Design review of the part built by this model. Coordinates are the model's own, in mm. Face numbers are marked on the shaded views. A direction names the side the tool comes from. Coordinates: 2 decimals unless noted, no trailing zeros. Loops run counter-clockwise (first coordinate to the right, second up) from the corner with the lowest first, then second, coordinate; pieces in that order, holes last. Notation, with made-up numbers: M 34,46 L 72,46 A24 cw 72,66 Z; hole C 61.25,-12 d10. An arc over 180 degrees is marked long. Put each result on its own line as item: value. Start each with the question number.
(1) For probe 1 along Z at (x, y) = (-14, -17.15); probe 2 along X at (y, z) = (-17.15, 0); probe 3 along X at (y, z) = (-19.5, -2.5), list the stretches that pass through material, from the lowest coordinate up. Write a range as [from, to].
(2) Take a section at D-D, the plane x = -5.5. Give the boundary of the cut face in (y, z), then the cut area to 3 significant figures.
(3) Clearance check with flat-ended pins moving along their axes: pin 1 (1.5 mm diameter, centred on x = 13, z = 2, fed in from +Y); pin 2 (1.6 mm diameter, centred on x = -14, z = 0, fed in from +Y); pin 3 (6.5 mm diameter, centred on y = -9.5, z = -0.5, fed in from -X); pin 4 (4 mm diameter, centred on y = -21, z = -1, fed in from +X). State where each tip first meets the part, or that it passes through.
(4) For the marked faces 1, 2, 3, 4 and 5, list the 3-axis set-ups (+Z, -Z, +X, -X, +Y, -Y) from which the entire face can be reached by the end or side of a thin tool; tool diameter is ignored.
(5) Take a section at C-C, the plane z = 2. Give the boundary of the cut face in (x, y).
(6) Take a section at B-B, the plane y = -16.25. Give the boundary of the cut face in (x, z), then the cut area to 3 significant figures.
(7) Take a section at A-A, the plane x = 14. Give the boundary of the cut face in (y, z).
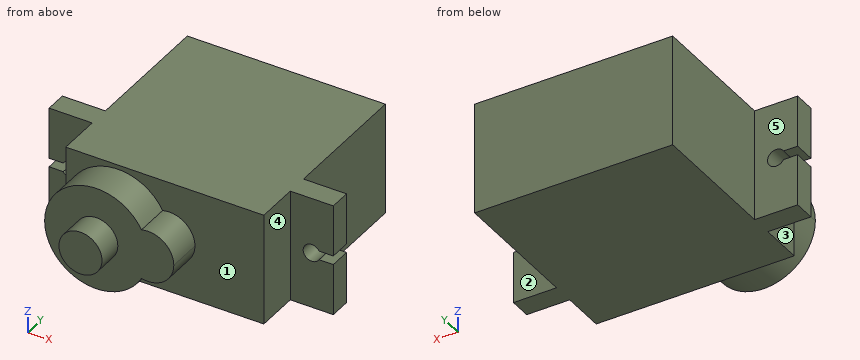
```python
from build123d import *

# Parameters (mm, degrees)
F0_R     = 2.5
F1_DEPTH = 23
F2_START = 15.5
F2_DEPTH = 2.5
F4_START = 23
F4_DEPTH = 4
F5_DEPTH = 30


with BuildPart() as f1:
    # F0 (on Front) → F1 (new body)
    with BuildSketch(Plane.XZ):
        Polygon((-11.5, -6.5), (11.5, -6.5), (11.5, 6.5), (-11.5, 6.5), (-11.5, 0), align=None)
        with BuildLine():
            ThreePointArc((-0.25, -2.9047375097), (-7, -5.8094750193), (-11.5, 0))
            ThreePointArc((-11.5, 0), (-7, 5.8094750193), (-0.25, 2.9047375097))
            ThreePointArc((-0.25, 2.9047375097), (2.3371173071, 2.3717082451), (3.5, 0))
            ThreePointArc((3.5, 0), (2.3371173071, -2.3717082451), (-0.25, -2.9047375097))
        make_face(mode=Mode.SUBTRACT)
        with BuildLine():
            ThreePointArc((3.5, 0), (2.3371173071, 2.3717082451), (-0.25, 2.9047375097))
            ThreePointArc((-0.25, 2.9047375097), (0.3094750193, 1.5), (0.5, 0))
            ThreePointArc((0.5, 0), (0.3094750193, -1.5), (-0.25, -2.9047375097))
            ThreePointArc((-0.25, -2.9047375097), (2.3371173071, -2.3717082451), (3.5, 0))
        make_face()
        with BuildLine():
            ThreePointArc((0.5, 0), (0.3094750193, 1.5), (-0.25, 2.9047375097))
            ThreePointArc((-0.25, 2.9047375097), (-2.5, 0), (-0.25, -2.9047375097))
            ThreePointArc((-0.25, -2.9047375097), (0.3094750193, -1.5), (0.5, 0))
        make_face()
        with BuildLine():
            ThreePointArc((-0.25, 2.9047375097), (-7, 5.8094750193), (-11.5, 0))
            ThreePointArc((-11.5, 0), (-7, -5.8094750193), (-0.25, -2.9047375097))
            ThreePointArc((-0.25, -2.9047375097), (-2.5, 0), (-0.25, 2.9047375097))
        make_face()
        with Locations((-5.5, 0)):
            Circle(F0_R, mode=Mode.SUBTRACT)
    extrude(amount=F1_DEPTH)

    # F0 (on Front) → F2 (join)
    with BuildSketch(Plane.XZ.offset(F2_START)):
        with BuildLine():
            Line((11.5, 6.5), (11.5, -6.5))
            Line((11.5, -6.5), (16.5, -6.5))
            Line((16.5, -6.5), (16.5, -0.5126835662))
            Line((16.5, -0.5126835662), (14.8585776383, -0.5126835662))
            ThreePointArc((14.8585776383, -0.5126835662), (13, 0), (14.8585776383, 0.5126835662))
            Line((14.8585776383, 0.5126835662), (16.5, 0.5126835662))
            Line((16.5, 0.5126835662), (16.5, 6.5))
            Line((16.5, 6.5), (11.5, 6.5))
        make_face()
    extrude(amount=F2_DEPTH)

    # F3: F1 across plane


with BuildPart() as f1_1:
    add(f1.part)
    add(f1.part.mirror(Plane.YZ))

    # F0 (on Front) → F4 (join)
    with BuildSketch(Plane.XZ.offset(F4_START)):
        with BuildLine():
            ThreePointArc((-0.25, 2.9047375097), (-7, 5.8094750193), (-11.5, 0))
            ThreePointArc((-11.5, 0), (-7, -5.8094750193), (-0.25, -2.9047375097))
            ThreePointArc((-0.25, -2.9047375097), (-2.5, 0), (-0.25, 2.9047375097))
        make_face()
        with Locations((-5.5, 0)):
            Circle(F0_R, mode=Mode.SUBTRACT)
        with BuildLine():
            ThreePointArc((3.5, 0), (2.3371173071, 2.3717082451), (-0.25, 2.9047375097))
            ThreePointArc((-0.25, 2.9047375097), (0.3094750193, 1.5), (0.5, 0))
            ThreePointArc((0.5, 0), (0.3094750193, -1.5), (-0.25, -2.9047375097))
            ThreePointArc((-0.25, -2.9047375097), (2.3371173071, -2.3717082451), (3.5, 0))
        make_face()
        with BuildLine():
            ThreePointArc((0.5, 0), (0.3094750193, 1.5), (-0.25, 2.9047375097))
            ThreePointArc((-0.25, 2.9047375097), (-2.5, 0), (-0.25, -2.9047375097))
            ThreePointArc((-0.25, -2.9047375097), (0.3094750193, -1.5), (0.5, 0))
        make_face()
    extrude(amount=F4_DEPTH)

    # F0 (on Front) → F5 (join)
    with BuildSketch(Plane.XZ):
        with Locations((-5.5, 0)):
            Circle(F0_R)
    extrude(amount=F5_DEPTH)


solid = f1_1.part
```
Computed values:
1. probe 1: z = [-6.5, -1], [1, 6.5]
1. probe 2: x = [-13, 13]
1. probe 3: x = [-11.5, 11.5]
2. outline: M -30,-2.5 L -27,-2.5 L -27,-6 L -23,-6 L -23,-6.5 L 0,-6.5 L 0,6.5 L -23,6.5 L -23,6 L -27,6 L -27,2.5 L -30,2.5 Z
2. area: 362 mm^2
3. pin 1: stops at y = -15.5
3. pin 2: passes through
3. pin 3: stops at x = -11.5
3. pin 4: stops at x = 11.5
4. face 1: -Y
4. face 2: +Z, -Z, +X, +Y
4. face 3: +Z, -Z, -X, -Y
4. face 4: +Z, -Z, +X, -Y
4. face 5: +Z, -Z, -X, +Y
5. outline: M -16.5,-18 L -11.5,-18 L -11.5,-23 L -11.16,-23 L -11.16,-27 L -7,-27 L -7,-30 L -4,-30 L -4,-27 L 2.74,-27 L 2.74,-23 L 11.5,-23 L 11.5,-18 L 16.5,-18 L 16.5,-15.5 L 11.5,-15.5 L 11.5,0 L -11.5,0 L -11.5,-15.5 L -16.5,-15.5 Z
6. outline: M -16.5,-6.5 L 16.5,-6.5 L 16.5,-0.51 L 14.86,-0.51 A1 cw long 14.86,0.51 L 16.5,0.51 L 16.5,6.5 L -16.5,6.5 L -16.5,0.51 L -14.86,0.51 A1 cw long -14.86,-0.51 L -16.5,-0.51 Z
6. area: 420 mm^2
7. outline: M -18,-6.5 L -15.5,-6.5 L -15.5,-1 L -18,-1 Z; M -18,1 L -15.5,1 L -15.5,6.5 L -18,6.5 Z
